Geometry: final body of the model. Coordinates: model frame, mm. Face numbers are marked on the shaded views. A direction names the side the tool comes from. Coordinates: 2 decimals unless noted, no trailing zeros. Loops run counter-clockwise (first coordinate to the right, second up) from the corner with the lowest first, then second, coordinate; pieces in that order, holes last. Notation, with made-up numbers: (66.5, 45) - (81.5, 45) arc R24 ccw to (81.5, 67) - close; hole circle Ø4 at (-1.75, -39). An arc over 180 degrees is marked (long way). Answer in a Markdown table with one row per item.
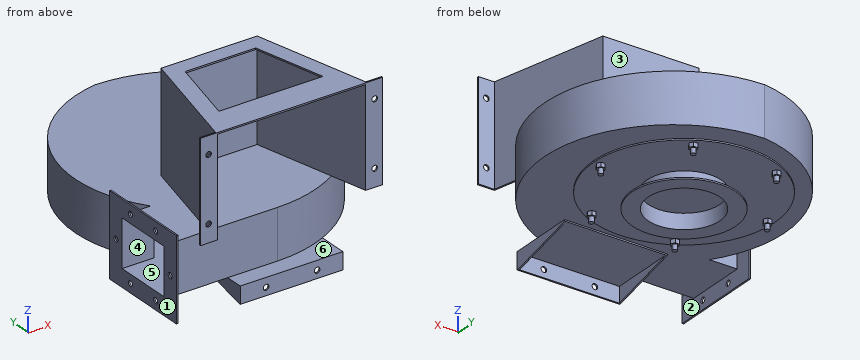
from build123d import *

# Parameters (mm, degrees)
SALIENTE_EXTRUIR1_DEPTH  = 170
SALIENTE_EXTRUIR2_DEPTH  = 2.5
CROQUIS4_R               = 4.7625
CORTAR_EXTRUIR1_DEPTH    = 2.5
SALIENTE_EXTRUIR3_DEPTH  = 2.5
SALIENTE_EXTRUIR4_DEPTH  = 80
SALIENTE_EXTRUIR5_DEPTH  = 2.5
CROQUIS8_W               = 140
CROQUIS8_H               = 161
CROQUIS8_W_2             = 80
CROQUIS8_H_2             = 101
SALIENTE_EXTRUIR6_DEPTH  = 2.5
CROQUIS9_R               = 4.7625
CORTAR_EXTRUIR2_DEPTH    = 2.5
CROQUIS10_R              = 61
CORTAR_EXTRUIR3_DEPTH    = 2.5
SALIENTE_EXTRUIR7_START  = 28.5
CROQUIS11_R              = 63.5
CROQUIS11_R_2            = 61
SALIENTE_EXTRUIR7_DEPTH  = 28.5
CROQUIS12_R              = 88
CROQUIS12_R_2            = 61
SALIENTE_EXTRUIR8_DEPTH  = 2.5
CROQUIS13_W              = 175
CROQUIS13_H              = 115
SALIENTE_EXTRUIR9_DEPTH  = 2.5
CROQUIS14_W              = 175
CROQUIS14_H              = 2.5
SALIENTE_EXTRUIR10_DEPTH = 26.5
SALIENTE_EXTRUIR11_DEPTH = 2.5
SALIENTE_EXTRUIR12_DEPTH = 2.5
CROQUIS17_R              = 4.7625
CORTAR_EXTRUIR4_DEPTH    = 2.5
CROQUIS18_R              = 154
SALIENTE_EXTRUIR13_DEPTH = 2.5
CROQUIS19_R              = 3.96875
SALIENTE_EXTRUIR14_DEPTH = 16
MATRIZC1_COUNT           = 6
CROQUIS20_R              = 3.96875
SALIENTE_EXTRUIR15_DEPTH = 7
MATRIZC3_COUNT           = 6
ESCALA1_SCALE            = 2


with BuildPart() as part:
    # Croquis1 → Saliente-Extruir1 (new body)
    with BuildSketch(Plane.XY):
        Polygon((0, 0), (29, 0), (75, 197), (235, 197), (281, 0), (310, 0), (310, 2.5), (282.983493442, 2.5), (236.983493442, 199.5), (73.016506558, 199.5), (27.016506558, 2.5), (0, 2.5), align=None)
    extrude(amount=SALIENTE_EXTRUIR1_DEPTH)

    # Croquis2 → Saliente-Extruir2 (add)
    with BuildSketch(Plane.XY.offset(170)):
        Polygon((29, 0), (281, 0), (269.286291687, 50.165229078), (235, 197), (75, 197), (40.713708313, 50.165229078), align=None)
        Polygon((243.652375223, 50), (66.347624777, 50), (94.834934422, 172), (215.165065578, 172), align=None, mode=Mode.SUBTRACT)
    extrude(amount=-SALIENTE_EXTRUIR2_DEPTH)

    # Croquis4 → Cortar-Extruir1 (cut)
    with BuildSketch(Plane(origin=(0, 2.5, 0), x_dir=(1, 0, 0), z_dir=(0, 1, 0))):
        with Locations(Location((13.508253279, -30, 0), (0, 0, 270))):
            Circle(CROQUIS4_R)
        with Locations(Location((13.508253279, -140, 0), (0, 0, 270))):
            Circle(CROQUIS4_R)
        with Locations(Location((296.491746721, -140, 0), (0, 0, 90))):
            Circle(CROQUIS4_R)
        with Locations(Location((296.491746721, -30, 0), (0, 0, 90))):
            Circle(CROQUIS4_R)
    extrude(amount=-CORTAR_EXTRUIR1_DEPTH, mode=Mode.SUBTRACT)

    # Croquis5 → Saliente-Extruir3 (add)
    with BuildSketch(Plane(origin=(0, 0, 0), x_dir=(-1, 0, 0), z_dir=(0, 0, -1))):
        with BuildLine():
            Line((0, 30), (40, 30))
            Line((40, 30), (40, 135))
            Line((40, 135), (-10, 135))
            ThreePointArc((-10, 135), (13.653759217, 342.621891967), (-152, 470))
            ThreePointArc((-152, 470), (-372, 250), (-152, 30))
            Line((-152, 30), (0, 30))
        make_face()
    extrude(amount=SALIENTE_EXTRUIR3_DEPTH)

    # Croquis6 → Saliente-Extruir4 (add)
    with BuildSketch(Plane(origin=(0, 0, -2.5), x_dir=(-1, 0, 0), z_dir=(0, 0, -1))):
        with BuildLine():
            Line((-10, 135), (40, 135))
            Line((40, 135), (40, 133))
            Line((40, 133), (38, 133))
            Line((38, 133), (-13.968512136, 133))
            ThreePointArc((-13.968512136, 133), (12.60152192, 339.954109112), (-152.141403753, 467.99995414))
            ThreePointArc((-152.141403753, 467.99995414), (-369.999988535, 249.92929812), (-152, 32))
            Line((-152, 32), (38, 32))
            Line((38, 32), (40, 32))
            Line((40, 32), (40, 30))
            Line((40, 30), (-152, 30))
            ThreePointArc((-152, 30), (-372, 250), (-152, 470))
            ThreePointArc((-152, 470), (13.653759217, 342.621891967), (-10, 135))
        make_face()
    extrude(amount=SALIENTE_EXTRUIR4_DEPTH)

    # Croquis7 → Saliente-Extruir5 (add)
    with BuildSketch(Plane(origin=(0, 0, -82.5), x_dir=(-1, 0, 0), z_dir=(0, 0, -1))):
        with BuildLine():
            Line((-10, 135), (40, 135))
            Line((40, 135), (40, 30))
            Line((40, 30), (-152, 30))
            ThreePointArc((-152, 30), (-372, 250), (-152, 470))
            ThreePointArc((-152, 470), (13.653759217, 342.621891967), (-10, 135))
        make_face()
    extrude(amount=SALIENTE_EXTRUIR5_DEPTH)

    # Croquis8 → Saliente-Extruir6 (add)
    with BuildSketch(Plane.ZY.offset(40)):
        with Locations((-42.5, 82.5)):
            Rectangle(CROQUIS8_W, CROQUIS8_H)
        with Locations((-42.5, 82.5)):
            Rectangle(CROQUIS8_W_2, CROQUIS8_H_2, mode=Mode.SUBTRACT)
    extrude(amount=-SALIENTE_EXTRUIR6_DEPTH)

    # Croquis9 → Cortar-Extruir2 (cut)
    with BuildSketch(Plane.ZY.offset(40)):
        with Locations((-42.5, 148)):
            Circle(CROQUIS9_R)
        with Locations((-97.5, 113)):
            Circle(CROQUIS9_R)
        with Locations((12.5, 113)):
            Circle(CROQUIS9_R)
        with Locations(Location((12.5, 52, 0), (0, 0, 180))):
            Circle(CROQUIS9_R)
        with Locations(Location((-97.5, 52, 0), (0, 0, 180))):
            Circle(CROQUIS9_R)
        with Locations(Location((-42.5, 17, 0), (0, 0, 180))):
            Circle(CROQUIS9_R)
    extrude(amount=-CORTAR_EXTRUIR2_DEPTH, mode=Mode.SUBTRACT)

    # Croquis10 → Cortar-Extruir3 (cut)
    with BuildSketch(Plane(origin=(0, 0, -85), x_dir=(-1, 0, 0), z_dir=(0, 0, -1))):
        with Locations((-155, 279.5)):
            Circle(CROQUIS10_R)
    extrude(amount=-CORTAR_EXTRUIR3_DEPTH, mode=Mode.SUBTRACT)

    # Croquis11 → Saliente-Extruir7 (add)
    with BuildSketch(Plane(origin=(0, 0, -85), x_dir=(-1, 0, 0), z_dir=(0, 0, -1)).offset(SALIENTE_EXTRUIR7_START)):
        with Locations(Location((-155, 279.5, 0), (0, 0, 180))):
            Circle(CROQUIS11_R)
        with Locations((-155, 279.5)):
            Circle(CROQUIS11_R_2, mode=Mode.SUBTRACT)
    extrude(amount=-SALIENTE_EXTRUIR7_DEPTH)

    # Croquis12 → Saliente-Extruir8 (add)
    with BuildSketch(Plane(origin=(0, 0, -113.5), x_dir=(-1, 0, 0), z_dir=(0, 0, -1))):
        with Locations((-155, 279.5)):
            Circle(CROQUIS12_R)
        with Locations((-155, 279.5)):
            Circle(CROQUIS12_R_2, mode=Mode.SUBTRACT)
    extrude(amount=-SALIENTE_EXTRUIR8_DEPTH)

    # Croquis13 → Saliente-Extruir9 (add)
    with BuildSketch(Plane(origin=(0, 0, -85), x_dir=(-1, 0, 0), z_dir=(0, 0, -1))):
        with Locations((-155, 57.5)):
            Rectangle(CROQUIS13_W, CROQUIS13_H)
    extrude(amount=SALIENTE_EXTRUIR9_DEPTH)

    # Croquis14 → Saliente-Extruir10 (add)
    with BuildSketch(Plane(origin=(0, 0, -87.5), x_dir=(-1, 0, 0), z_dir=(0, 0, -1))):
        with Locations((-155, 1.25)):
            Rectangle(CROQUIS14_W, CROQUIS14_H)
    extrude(amount=SALIENTE_EXTRUIR10_DEPTH)

    # Croquis15 → Saliente-Extruir11 (add)
    with BuildSketch(Plane.ZY.offset(-67.5)):
        Polygon((-114, 2.5), (-87.5, 115), (-85, 115), (-85, 0), (-114, 0), align=None)
    extrude(amount=-SALIENTE_EXTRUIR11_DEPTH)

    # Croquis16 → Saliente-Extruir12 (add)
    with BuildSketch(Plane(origin=(242.5, 0, 0), x_dir=(0, 0, -1), z_dir=(1, 0, 0))):
        Polygon((114, 2.5), (87.5, 115), (85, 115), (85, 0), (114, 0), align=None)
    extrude(amount=-SALIENTE_EXTRUIR12_DEPTH)

    # Croquis17 → Cortar-Extruir4 (cut)
    with BuildSketch(Plane.XZ):
        with Locations(Location((198.5, -100.75, 0), (0, 0, 270))):
            Circle(CROQUIS17_R)
        with Locations(Location((111.5, -100.75, 0), (0, 0, 270))):
            Circle(CROQUIS17_R)
    extrude(amount=-CORTAR_EXTRUIR4_DEPTH, mode=Mode.SUBTRACT)

    # Croquis18 → Saliente-Extruir13 (add)
    with BuildSketch(Plane(origin=(0, 0, -85), x_dir=(-1, 0, 0), z_dir=(0, 0, -1))):
        with Locations(Location((-155, 279.5, 0), (0, 0, 180))):
            Circle(CROQUIS18_R)
    extrude(amount=SALIENTE_EXTRUIR13_DEPTH)

    # Croquis19 → Saliente-Extruir14 (add)
    with BuildSketch(Plane(origin=(0, 0, -87.5), x_dir=(-1, 0, 0), z_dir=(0, 0, -1))):
        with Locations((-13, 279.5)):
            Circle(CROQUIS19_R)
    saliente_extruir14 = extrude(amount=SALIENTE_EXTRUIR14_DEPTH)

    # MatrizC1: Saliente-Extruir14 ×6 about axis
    matrizc1_axis = Axis((155, 279.5, 0), (0, 0, 1))
    for i in range(1, MATRIZC1_COUNT):
        add(saliente_extruir14.rotate(matrizc1_axis, i * 360 / MATRIZC1_COUNT))

    # Croquis20 → Saliente-Extruir15 (add)
    with BuildSketch(Plane(origin=(0, 0, -87.5), x_dir=(-1, 0, 0), z_dir=(0, 0, -1))):
        Polygon((-6.07179677, 279.5), (-9.535898385, 285.5), (-16.464101615, 285.5), (-19.92820323, 279.5), (-16.464101615, 273.5), (-9.535898385, 273.5), align=None)
        with Locations((-13, 279.5)):
            Circle(CROQUIS20_R, mode=Mode.SUBTRACT)
    saliente_extruir15 = extrude(amount=SALIENTE_EXTRUIR15_DEPTH)

    # MatrizC3: Saliente-Extruir15 ×6 about axis
    matrizc3_axis = Axis((155, 279.5, 0), (0, 0, 1))
    for i in range(1, MATRIZC3_COUNT):
        add(saliente_extruir15.rotate(matrizc3_axis, i * 360 / MATRIZC3_COUNT))


with BuildPart() as part_1:
    # Escala1: scaled about (153.867838304, 207.115658643, -22.79882081)
    add(part.part.scale(ESCALA1_SCALE).moved(Location((-153.867838304, -207.115658643, 22.79882081))))


solid = part_1.part
(1) Cut plane B-B on x = 490. Output: boundary loops of the cut face in (y, z).
Verdict:
| item | result |
|---|---|
| outline | (13.44, -147.2) - (572.33, -147.2) - (572.33, 22.8) - (13.44, 22.8) - close; hole (19.78, -142.2) - (565.99, -142.2) - (565.99, 17.8) - (19.78, 17.8) - close |
(2) Ray query, probe 1 along Z at (x, y) = (41, 222); probe 2 along Y at (x, z) = (16, -170.5); probe 3 along Z at (x, y) = (319, 265). Return the intervals inside material, ascending.
Verdict:
| item | result |
|---|---|
| probe 1 | z = -204.2 to -199.2, -152.2 to -142.2, 17.8 to 22.8 |
| probe 2 | y = -207.12 to -202.12, 98.22 to 113.65, 590.12 to 605.55 |
| probe 3 | z = -152.2 to -142.2, 17.8 to 22.8 |
(3) Cut plane A-A on z = 191.5. Output: boundary loops of the cut face in (x, y).
Verdict:
| item | result |
|---|---|
| outline | (-153.87, -207.12) - (-95.87, -207.12) - (-3.87, 186.88) - (316.13, 186.88) - (408.13, -207.12) - (466.13, -207.12) - (466.13, -202.12) - (412.1, -202.12) - (320.1, 191.88) - (-7.83, 191.88) - (-99.83, -202.12) - (-153.87, -202.12) - close |
(4) First-contact query: pin 1 Ø5 at (y, z) = (389.5, -11.5) entering from -X; pin 2 Ø16 at (x, z) = (-121.5, 152.5) entering from +Y; pin 3 Ø1 at (x, y) = (378.5, 317) entering from -Z. Flat tips, straight axial feed; report the tip coordinate or a pass-through.
Verdict:
| item | result |
|---|---|
| pin 1 | stops at x = -208.25 |
| pin 2 | stops at y = -202.12 |
| pin 3 | stops at z = -152.2 |
(5) Access query for the marked faces 4, 5 and 6. Directions: +Z, -Z, +X, -X, +Y, -Y. A direction counts if a zero-diameter tool reaches every point of the face in a straight line with its end or side. Return the directions, or none.
Verdict:
| item | result |
|---|---|
| face 4 | -X |
| face 5 | none |
| face 6 | +X, -Y |
(6) Cut plane C-C on y = 376. Output: boundary loops of the cut face in (x, z).
Verdict:
| item | result |
|---|---|
| outline | (-210.06, -147.2) - (-150.92, -147.2) - (-150.92, -152.2) - (31.44, -152.2) - (31.44, -199.2) - (-18.21, -199.2) - (-18.21, -204.2) - (36.54, -204.2) - (36.54, -152.2) - (275.72, -152.2) - (275.72, -204.2) - (330.47, -204.2) - (330.47, -199.2) - (280.82, -199.2) - (280.82, -152.2) - (463.19, -152.2) - (463.19, -147.2) - (582.21, -147.2) - (582.21, 22.8) - (-210.06, 22.8) - close; hole (-206.02, -142.2) - (36.54, -142.2) - (36.54, -147.2) - (275.72, -147.2) - (275.72, -142.2) - (578.14, -142.2) - (578.14, 17.8) - (-206.02, 17.8) - close |
(7) Pull-direction query (X, two-part tool) for the marked faces 1, 2 and 3; classes: pulls with the +X half, pulls with the -X half, needs draft (parallel to the pull), parting line crosses it, or undercut.
Verdict:
| item | result |
|---|---|
| face 1 | pulls with the -X half |
| face 2 | undercut |
| face 3 | needs draft |
